Geometry check sheet. Reference: the model listing, model coordinates, mm. A direction names the side the tool comes from. Round coordinates to 2 decimals unless told otherwise and drop trailing zeros. Loops run counter-clockwise (first coordinate to the right, second up) from the corner with the lowest first, then second, coordinate; pieces in that order, holes last.
Autodesk Inventor part; units mm, degrees
ref_plane "YZ Plane" through (0, 0, 0) normal (1, 0, 0) x (0, 1, 0)
ref_plane "XZ Plane" through (0, 0, 0) normal (0, 1, 0) x (-1, 0, 0)
ref_plane "XY Plane" through (0, 0, 0) normal (0, 0, 1) x (1, 0, 0)
sketch "Sketch1" plane through (0, 0, 0) normal (0, 0, 1) x (1, 0, 0)
  line L0 (6.35, 0) -> (57.15, 0)
  line L1 (63.5, 6.35) -> (63.5, 82.55)
  line L2 (57.15, 88.9) -> (6.35, 88.9)
  line L3 (0, 82.55) -> (0, 6.35)
  arc A0 (6.35, 88.9) -> (0, 82.55) centre (6.35, 82.55) ccw
  arc A1 (63.5, 82.55) -> (57.15, 88.9) centre (57.15, 82.55) ccw
  arc A2 (57.15, 0) -> (63.5, 6.35) centre (57.15, 6.35) ccw
  arc A3 (0, 6.35) -> (6.35, 0) centre (6.35, 6.35) ccw
  point P0 (0, 0)
  point P1 (63.5, 88.9)
  point P2 (63.5, 0)
  point P3 (0, 88.9)
  dimension "d0" = 88.9
  dimension "d1" = 63.5
  dimension "d2" = 6.35
extrude "Extrusion1" add sketch "Sketch1" along normal blind 25.4
sketch "Sketch2" plane through (6.35, 88.9, 0) normal (0, 1, 0) x (1, 0, 0)
  line L0 (6.35, -2.032) -> (16.002, -2.032)
  line L1 (16.002, -2.032) -> (16.002, -5.334)
  line L2 (16.002, -5.334) -> (6.35, -5.334)
  line L3 (6.35, -5.334) -> (6.35, -2.032)
  line L4 (0, 0) -> (0, -25.4)
  line L5 (50.8, 0) -> (0, 0)
  line L6 (28.702, -5.334) -> (19.05, -5.334)
  line L7 (19.05, -2.032) -> (28.702, -2.032)
  line L8 (28.702, -2.032) -> (28.702, -5.334)
  line L9 (19.05, -5.334) -> (19.05, -2.032)
  line L10 (16.002, -10.414) -> (6.35, -10.414)
  line L11 (6.35, -7.112) -> (16.002, -7.112)
  line L12 (16.002, -7.112) -> (16.002, -10.414)
  line L13 (6.35, -10.414) -> (6.35, -7.112)
  line L14 (28.702, -10.414) -> (19.05, -10.414)
  line L15 (19.05, -7.112) -> (28.702, -7.112)
  line L16 (28.702, -7.112) -> (28.702, -10.414)
  line L17 (19.05, -10.414) -> (19.05, -7.112)
  line L18 (33.02, -2.032) -> (42.672, -2.032)
  line L19 (42.672, -2.032) -> (42.672, -10.414)
  line L20 (42.672, -10.414) -> (33.02, -10.414)
  line L21 (33.02, -10.414) -> (33.02, -2.032)
  point P0 (-6.35, 0)
  point P1 (6.35, -3.683)
  point P2 (19.05, -3.683)
  point P3 (6.35, -8.763)
  point P4 (19.05, -8.763)
  point P5 (37.846, -2.032)
  dimension "d5" = 6.35
  dimension "d6" = 9.652
  dimension "d7" = 3.302
  dimension "d8" = 2.032
  dimension "d11" = 12.7
  dimension "d14" = 5.08
  dimension "d17" = 8.382
  dimension "d18" = 9.652
  dimension "d19" = 4.318
  dimension "d20" = 0
extrude "Extrusion2" cut sketch "Sketch2" against normal blind 10.16
sketch "Sketch3" plane through (0, 6.35, 0) normal (-1, 0, 0) x (0, 0, 1)
  line L0 (12.7, 10.16) -> (12.7, 15.24) construction
  line L1 (12.065, 10.16) -> (12.065, 15.24)
  line L2 (13.335, 15.24) -> (13.335, 10.16)
  arc A0 (12.065, 10.16) -> (13.335, 10.16) centre (12.7, 10.16) ccw
  arc A1 (13.335, 15.24) -> (12.065, 15.24) centre (12.7, 15.24) ccw
  line L3 (25.4, 76.2) -> (25.4, 0)
  line L4 (0, 0) -> (25.4, 0)
  line L5 (13.335, 27.94) -> (13.335, 22.86)
  arc A2 (12.065, 22.86) -> (13.335, 22.86) centre (12.7, 22.86) ccw
  line L6 (12.065, 22.86) -> (12.065, 27.94)
  arc A3 (13.335, 27.94) -> (12.065, 27.94) centre (12.7, 27.94) ccw
  line L7 (13.335, 40.64) -> (13.335, 35.56)
  arc A4 (12.065, 35.56) -> (13.335, 35.56) centre (12.7, 35.56) ccw
  line L8 (12.065, 35.56) -> (12.065, 40.64)
  arc A5 (13.335, 40.64) -> (12.065, 40.64) centre (12.7, 40.64) ccw
  circle A6 centre (12.7, 50.8) radius 2.286
  line L9 (0, 76.2) -> (25.4, 76.2)
  point P0 (0, -6.35)
  point P1 (12.7, 12.7)
  point P2 (12.7, 76.2)
  dimension "d23" = 5.08
  dimension "d24" = 0.635
  dimension "d25" = 12.7
  dimension "d26" = 12.7
  dimension "d29" = 12.7
  dimension "d34" = 4.572
  dimension "d35" = 12.7
  dimension "d36" = 25.4
extrude "Extrusion3" cut sketch "Sketch3" against normal blind 10.16
properties part number "RaspberryPi"
1) Sectioned sample at A-A, the plane x = 28.5. Record the cut outline in (y, z).
Report:
outline: (0, 0) - (88.9, 0) - (88.9, 2.03) - (78.74, 2.03) - (78.74, 5.33) - (88.9, 5.33) - (88.9, 7.11) - (78.74, 7.11) - (78.74, 10.41) - (88.9, 10.41) - (88.9, 25.4) - (0, 25.4) - close
2) Mould release check, pull along Y, two halves, no side actions. Record for faces 1 (the face through (5.009, 59.417, 12.402)), 2 (the face through (18, 84, 5.334)), 3 (the face through (61.59, 87.09, 12.52)): +Y half, -Y half, draft (parallel to the pull), parting line (faces both ways), or undercut.
Report:
face 1: undercut
face 2: draft
face 3: +Y half
3) Gauge pin test, flat ends, axial feed: pin 1 (1.7 mm diameter, centred on y = 85, z = 4, fed in from -X); pin 2 (2.5 mm diameter, centred on y = 84.5, z = 9.5, fed in from -X); pin 3 (1 mm diameter, centred on x = 28, z = 4.5, fed in from +Y). Record the tip position at first contact, or that the pin passes through.
Report:
pin 1: stops at x = 0.2
pin 2: stops at x = 0.04
pin 3: stops at y = 78.74
4) Access from +Z, -Z, +X, -X, +Y, -Y to the whole of each face (thin tool, end or side, straight path). Record for faces 4 (the face through (22.352, 84, 9)), 5 (the face through (5, 19, 13.335)), 6 (the face through (31, 45, 25.4)).
Report:
face 4: +Y
face 5: -X
face 6: +Z, +X, -X, +Y, -Y
5) Sectioned sample at C-C, the plane x = 4.5. Record the cut outline in (y, z) (3 decimals).
Report:
outline: (0.275, 0) - (88.625, 0) - (88.625, 25.4) - (0.275, 25.4) - close; hole (16.51, 12.065) - (21.59, 12.065) arc R0.635 ccw to (21.59, 13.335) - (16.51, 13.335) arc R0.635 ccw to start; hole (29.21, 12.065) - (34.29, 12.065) arc R0.635 ccw to (34.29, 13.335) - (29.21, 13.335) arc R0.635 ccw to start; hole (41.91, 12.065) - (46.99, 12.065) arc R0.635 ccw to (46.99, 13.335) - (41.91, 13.335) arc R0.635 ccw to start; hole circle Ø4.572 at (57.15, 12.7)
6) Scan lines: line 1 along X through (y, z) = (79.5, 2.75); line 2 along Y through (x, z) = (8, 12.7) (3 decimals); line 3 along Z through (x, y) = (7, 57). Record each from-to range of solid material in increasing order.
Report:
line 1: x = 0 to 12.7, 22.35 to 25.4, 35.05 to 39.37, 49.02 to 63.5
line 2: y = 0 to 15.875, 22.225 to 28.575, 34.925 to 41.275, 47.625 to 54.864, 59.436 to 88.9
line 3: z = 0 to 10.42, 14.98 to 25.4
7) Sectioned sample at B-B, the plane y = 57.15. Record the cut outline in (x, z).
Report:
outline: (0, 0) - (63.5, 0) - (63.5, 25.4) - (0, 25.4) - (0, 14.99) - (10.16, 14.99) - (10.16, 10.41) - (0, 10.41) - close
